Input: part model. Units: mm. Frame: model coordinates. A direction names the side the tool comes from. Round coordinates to 2 decimals unless told otherwise and drop trailing zeros. Write each loop counter-clockwise with the first axis right and the second up, starting at its lowest first coordinate (ties: lowest second). Pieces come first, ordered by that corner, then holes. Notation, with made-up numbers: (85, 75.25) -> (107, 75.25) arc R9 cw to (107, 83.25) -> close; hole circle Ø2 at (9, -24.75). An arc over 180 degrees is marked (long way). Use CSV: the item, a comma, the result in double quotes.
Autodesk Inventor part; units mm, degrees
ref_plane "YZ Plane" through (0, 0, 0) normal (1, 0, 0) x (0, 1, 0)
ref_plane "XZ Plane" through (0, 0, 0) normal (0, 1, 0) x (-1, 0, 0)
ref_plane "XY Plane" through (0, 0, 0) normal (0, 0, 1) x (1, 0, 0)
sketch "Sketch2" plane through (0, 0, 0) normal (1, 0, 0) x (0, 1, 0)
  line L0 (12, 15.675) -> (-12, 15.675)
  line L1 (-12, 15.675) -> (-12, -15.675)
  line L2 (-12, -15.675) -> (12, -15.675)
  line L3 (12, -15.675) -> (12, 15.675)
  point P0 (0, 0)
  dimension "d4" = 24
  dimension "d5" = 31.35
  dimension "d6" = 15.675
  dimension "d7" = 12
extrude "Extrusion1" add sketch "Sketch2" along normal blind 3.175
sketch "Sketch3" plane through (3.175, 0, 0) normal (1, 0, 0) x (0, 0, -1)
  line L0 (-15.675, -12) -> (15.675, -12)
  line L1 (-10.4, -12) -> (10.4, -12)
  line L2 (10.4, -12) -> (10.4, -6.5)
  line L3 (10.4, -6.5) -> (-10.4, -6.5)
  line L4 (-10.4, -6.5) -> (-10.4, -12)
  point P0 (0, 0)
  dimension "d16" = 20.8
  dimension "d17" = 10.4
  dimension "d18" = 5.5
extrude "Extrusion2" cut sketch "Sketch3" against normal blind 2.4
sketch "Sketch4" plane through (3.175, 0, 0) normal (1, 0, 0) x (0, 0, -1)
  line L0 (-8.85, 10) -> (8.85, 10)
  line L1 (8.85, 10) -> (8.85, -1.6)
  line L2 (8.85, -1.6) -> (-8.85, -1.6)
  line L3 (-8.85, -1.6) -> (-8.85, 10)
  line L4 (-10.4, -6.5) -> (10.4, -6.5)
  line L5 (10.4, -12) -> (-10.4, -12)
  point P0 (0, 4.2)
  dimension "d21" = 17.7
  dimension "d22" = 8.85
  dimension "d23" = 5.8
  dimension "d24" = 11.6
  dimension "d27" = 10.4
extrude "Extrusion3" cut sketch "Sketch4" against normal blind 1.3
sketch "Sketch5" plane through (3.175, 0, 0) normal (1, 0, 0) x (0, 0, -1)
  circle A0 centre (-10.65, 10.9) radius 0.8411
  circle A1 centre (10.65, 10.9) radius 0.8411
  line L0 (-15.675, 12) -> (-15.675, -12)
  line L1 (15.675, 12) -> (-15.675, 12)
  line L2 (15.675, -12) -> (15.675, 12)
  line L3 (8.85, 10) -> (8.85, -1.6)
  line L4 (-8.85, 10) -> (8.85, 10)
  point P0 (0, 0)
  dimension "d31" = 1.6822
  dimension "d33" = 1.6822
  dimension "d60" = 1.8
  dimension "d62" = 0.9
  dimension "d67" = 0.9
  dimension "d68" = 1.8
extrude "Extrusion7" [suppressed]
sketch "Sketch12" plane through (0, 12, 15.675) normal (0, 1, 0) x (1, 0, 0)
  line L0 (0, 31.35) -> (0, 0)
  line L1 (0, 0) -> (3.175, 0)
  line L2 (3.175, 31.35) -> (3.175, 0)
  line L3 (0, 31.35) -> (3.175, 31.35)
  point P0 (0, 15.675)
extrude "Extrusion14" add sketch "Sketch12" along normal blind 11.43
sketch "Sketch13" plane through (0, 0, 0) normal (-1, 0, 0) x (0, 0, 1)
  circle A0 centre (-6.3786, 20.89) radius 1.4224
  circle A1 centre (6.3786, 20.89) radius 1.4224
  line L0 (-15.675, 23.43) -> (15.675, 23.43)
  line L1 (-15.675, -12) -> (-15.675, 23.43)
  line L2 (15.675, 23.43) -> (15.675, -12)
  circle A2 centre (0, 15.175) radius 1.4224
  point P0 (0, 0)
  dimension "d92" = 2.8448
  dimension "d93" = 2.8448
  dimension "d94" = 2.54
  dimension "d95" = 9.2964
  dimension "d96" = 9.2964
  dimension "d97" = 2.54
  dimension "d98" = 2.8448
  dimension "d99" = 8.255
  dimension "d100" = 31.35
  dimension "d101" = 15.675
extrude "Extrusion15" cut sketch "Sketch13" against normal through all
sketch "Sketch14" plane through (3.175, 0, 0) normal (1, 0, 0) x (0, 0, -1)
  circle A0 centre (12.65, -2.5) radius 1.05
  line L0 (10.4, -12) -> (15.675, -12)
  line L1 (15.675, -12) -> (15.675, -0.0588)
  circle A1 centre (12.65, 10) radius 1.05
  line L2 (15.675, -12) -> (15.675, 23.43)
  line L3 (10.4, -6.5) -> (10.4, -12)
  line L4 (-15.675, 23.43) -> (15.675, 23.43)
  line L5 (0, 23.43) -> (0, -12) construction
  line L6 (-15.675, -12) -> (15.675, -12)
  circle A2 centre (-12.65, -2.5) radius 1.05
  circle A3 centre (-12.65, 10) radius 1.05
  point P0 (0, 0)
  point P1 (15.675, 6.4088)
  dimension "d105" = 9.5
  dimension "d108" = 12.5
  dimension "d111" = 2.25
  dimension "d112" = 2.25
extrude "Extrusion16" [suppressed]
sketch "Sketch15" plane through (0, 0, 0) normal (-1, 0, 0) x (0, 0, 1)
  circle A0 centre (-11.0465, 10) radius 1.05
  line L0 (-15.675, -12) -> (-15.675, 23.43)
  line L1 (-15.675, 23.43) -> (15.675, 23.43)
  line L2 (0, -12) -> (0, 23.43) construction
  line L3 (15.675, 23.43) -> (-15.675, 23.43)
  circle A1 centre (11.0465, 10) radius 1.05
  circle A2 centre (-10.5016, -2.4993) radius 1.05
  circle A3 centre (10.5016, -2.4993) radius 1.05
  point P0 (0, 0)
  dimension "d115" = 2.1
  dimension "d117" = 13.43
  dimension "d125" = 11.0465
  dimension "d128" = 2.1
  dimension "d129" = 2.1
  dimension "d130" = 2.1
  dimension "d131" = 22.0929
  dimension "d132" = 21.0033
  dimension "d133" = 12.4993
  dimension "d134" = 10.5016
  dimension "d135" = 12.4993
extrude "Extrusion17" [suppressed]
sketch "Sketch16" plane through (3.175, 0, 0) normal (1, 0, 0) x (0, 0, -1)
  circle A0 centre (-10.35, 10) radius 1.05
  circle A1 centre (10.65, 10) radius 1.05
  circle A2 centre (10.65, -2.5) radius 1.05
  circle A3 centre (-10.35, -2.5) radius 1.05
  point P0 (0, 0)
extrude "Extrusion18" cut sketch "Sketch16" against normal through all
sketch "Sketch17" plane through (3.175, 0, 0) normal (1, 0, 0) x (0, 0, -1)
  line L0 (-15.675, -12) -> (15.675, -12)
  line L1 (-13.575, -12) -> (13.575, -12)
  line L2 (13.575, -12) -> (13.575, -6.5)
  line L3 (13.575, -6.5) -> (-13.575, -6.5)
  line L4 (-13.575, -6.5) -> (-13.575, -12)
  line L5 (-10.4, -6.5) -> (10.4, -6.5)
  line L6 (10.4, -6.5) -> (10.4, -12)
  line L7 (-10.4, -12) -> (-10.4, -6.5)
  point P0 (0, 0)
  dimension "d138" = 0
  dimension "d139" = 3.175
  dimension "d140" = 3.175
extrude "Extrusion19" cut sketch "Sketch17" against normal blind 2.3876 contours L4 L3 L7 L0 | L6 L3 L2 L0
sketch "Sketch18" plane through (3.175, 0, 0) normal (1, 0, 0) x (0, 0, -1)
  circle A0 centre (-10.35, 10) radius 1.05
  circle A1 centre (10.65, 10) radius 1.05
  circle A2 centre (10.65, -2.5) radius 1.05
  circle A3 centre (-10.35, -2.5) radius 1.05
  arc A4 (-9.0198, 8.4192) -> (-8.284, 10) centre (-10.35, 10) ccw
  arc A5 (8.584, 10) -> (9.3198, 8.4192) centre (10.65, 10) ccw
  arc A6 (9.5482, -0.7523) -> (10.65, -4.566) centre (10.65, -2.5) ccw
  arc A7 (-10.35, -4.566) -> (-9.2482, -0.7523) centre (-10.35, -2.5) ccw
  line L0 (-12.5392, 5.1935) -> (-12.4941, 2.372)
  line L1 (13.569, 2.4227) -> (13.569, 5.2442)
  line L2 (5.409, 13.3584) -> (-5.109, 13.3584)
  line L3 (-10.35, -4.566) -> (-10.35, -6.5)
  line L4 (-10.35, -6.5) -> (10.65, -6.5)
  line L5 (-13.575, -6.5) -> (13.575, -6.5)
  line L6 (10.65, -4.566) -> (10.65, -6.5)
  line L7 (9.5482, -0.7523) -> (10.394, -0.7523)
  line L8 (9.3198, 8.4192) -> (10.394, 8.4192)
  line L9 (8.584, 10) -> (8.584, 10.1834)
  line L10 (-8.284, 10) -> (-8.284, 10.1834)
  line L11 (-9.0198, 8.4192) -> (-9.3646, 8.4192)
  line L12 (-9.2482, -0.7523) -> (-9.3195, -0.7523)
  arc A8 (13.569, 5.2442) -> (10.394, 8.4192) centre (10.394, 5.2442) ccw
  arc A9 (8.584, 10.1834) -> (5.409, 13.3584) centre (5.409, 10.1834) ccw
  arc A10 (-5.109, 13.3584) -> (-8.284, 10.1834) centre (-5.109, 10.1834) ccw
  arc A11 (-9.3646, 8.4192) -> (-12.5392, 5.1935) centre (-9.3646, 5.2442) ccw
  arc A12 (-12.4941, 2.372) -> (-9.3195, -0.7523) centre (-9.3195, 2.4227) ccw
  arc A13 (10.394, -0.7523) -> (13.569, 2.4227) centre (10.394, 2.4227) ccw
  point P0 (0, 0)
  point P1 (-12.4442, -0.7523)
  point P2 (-12.5907, 8.4192)
  dimension "d143" = 1.016
  dimension "d144" = 1.016
  dimension "d145" = 1.016
  dimension "d146" = 1.016
  dimension "d147" = 3.175
extrude "Extrusion20" cut sketch "Sketch18" against normal blind 2.159 contours A4 L10 A10 L2 A9 L9 A5 L8 A8 L1 A13 L7 A6 L6 L4 L3 A7 L12 A12 L0 A11 L11
sketch "Sketch19" plane through (3.175, 0, 0) normal (1, 0, 0) x (0, 0, -1)
  line L0 (-13.575, -12) -> (-13.575, -6.5)
  line L1 (-13.575, -12) -> (13.7056, -12)
  line L2 (13.7056, -12) -> (13.7056, -9.675)
  line L3 (10.5306, -6.5) -> (-10.4, -6.5)
  line L4 (-13.575, -9.675) -> (-13.575, -12)
  arc A0 (-10.4, -6.5) -> (-13.575, -9.675) centre (-10.4, -9.675) ccw
  arc A1 (13.7056, -9.675) -> (10.5306, -6.5) centre (10.5306, -9.675) ccw
  point P0 (0, 0)
  dimension "d150" = 3.175
fillet "Fillet1" radius 3.175 2 edges at (1.9812, -6.5, -13.575) (1.9812, -6.5, 13.575)
equation "\"d31\" = d30"
equation "\"d33\" = d30"
equation "\"d67\" = d62"
equation "\"d68\" = d60"
equation "\"d93\" = d92"
equation "\"d96\" = d95"
equation "\"d98\" = d92"
equation "\"d101\" = 0.5 * d100"
equation "\"d112\" = d111"
equation "\"d125\" = 0.5 * d131"
equation "\"d128\" = d115"
equation "\"d129\" = d115"
equation "\"d130\" = d115"
equation "\"d134\" = 0.5 * d132"
equation "\"d135\" = d133"
properties part number "Pi cCam Mount" material "Aluminum 6061-AHC"
Item 1: Section query B-B on z = 0. Return the cut outline in (x, y) (3 decimals), plus the area to 3 significant figures.
Worked answers:
outline,"(0, -12) -> (0.775, -12) -> (0.775, -6.5) -> (1.016, -6.5) -> (1.016, 13.358) -> (3.175, 13.358) -> (3.175, 13.753) -> (0, 13.753) -> close; (0, 16.597) -> (3.175, 16.597) -> (3.175, 23.43) -> (0, 23.43) -> close"
area,"47.4 mm²"
Item 2: Section query C-C on y = 7. Return the cut outline in (x, z) (3 decimals).
Worked answers:
outline,"(0, -15.675) -> (3.175, -15.675) -> (3.175, -13.039) -> (1.016, -13.039) -> (1.016, 12.01) -> (3.175, 12.01) -> (3.175, 15.675) -> (0, 15.675) -> close"
Item 3: Section query D-D on z = 7. Return the cut outline in (x, y) (3 decimals), plus the area to 3 significant figures.
Worked answers:
outline,"(0, -12) -> (0.775, -12) -> (0.775, -6.5) -> (1.016, -6.5) -> (1.016, 12.734) -> (3.175, 12.734) -> (3.175, 19.611) -> (0, 19.611) -> close; (0, 22.169) -> (3.175, 22.169) -> (3.175, 23.43) -> (0, 23.43) -> close"
area,"49.6 mm²"
Item 4: First-contact query: pin 1 Ø1 at (y, z) = (7.5, 6) entering from +X; pin 2 Ø1.6 at (y, z) = (-9.5, -2) entering from +X (3 decimals). Flat tips, straight axial feed; report the tip coordinate or a pass-through.
Worked answers:
pin 1,"stops at x = 1.02"
pin 2,"stops at x = 0.775"
Item 5: Pull-direction query (Z, two-part tool) for faces 4 (the face through (2.111, 0.184, 11.571)), 5 (the face through (2, 5, 15.675)), 6 (the face through (0, 5, 0)); classes: +Z half, -Z half, draft (parallel to the pull), parting line (faces both ways), or undercut.
Worked answers:
face 4,"undercut"
face 5,"+Z half"
face 6,"draft"
Item 6: Section query A-A on y = -2.5. Return the cut outline in (x, z) (3 decimals).
Worked answers:
outline,"(0, -15.675) -> (3.175, -15.675) -> (3.175, -11.7) -> (0, -11.7) -> close; (0, -9.6) -> (3.175, -9.6) -> (3.175, -8.584) -> (1.016, -8.584) -> (1.016, 8.284) -> (3.175, 8.284) -> (3.175, 9.3) -> (0, 9.3) -> close; (0, 11.4) -> (3.175, 11.4) -> (3.175, 15.675) -> (0, 15.675) -> close"
Item 7: Set-up query: faces 1 (the face through (2, -6, -10.65)), 2 (the face through (1.6, -2.5, 11.4)), 3 (the face through (2.111, -3.037, -8.655)). Return all of +Z, -Z, +X, -X, +Y, -Y with unobstructed straight access to the full face (end or side cutting, diameter ignored); none if empty.
Worked answers:
face 1,"+X, -Y"
face 2,"+X, -X"
face 3,"+X"
Item 8: Line query: line 1 (Z direction, x = 1.2, y = -11) (3 decimals); line 2 (Y direction, x = 1.7, z = 0); line 3 (Z direction, x = 1.2, y = 3) (3 decimals). Output: solid intervals per line, ascending.
Worked answers:
line 1,"z = -15.675 to -13.575, 13.575 to 15.675"
line 2,"y = 13.36 to 13.75, 16.6 to 23.43"
line 3,"z = -15.675 to -13.569, 12.504 to 15.675"
